Check sheet for the modelled part. Datum: model origin and axes. Units: mm. A direction names the side the tool comes from. Round coordinates to 2 decimals unless told otherwise and drop trailing zeros. Write each loop counter-clockwise with the first axis right and the second up, starting at its lowest first coordinate (ties: lowest second). Pieces come first, ordered by that corner, then holes. Notation, with made-up numbers: (-27, 9.25) -> (23, 9.25) arc R32 ccw to (23, 38.25) -> close; hole circle Ø5 at (87, 73.5). An arc over 180 degrees is marked (long way). Answer as a JSON object with one key per item and string values. Group by question number.
```python
from build123d import *

# Parameters (mm, degrees)
SCHIZZO1_R                   = 3
ESTRUSIONE_ESTRUSIONE1_DEPTH = 14
SMUSSO1_SIZE                 = 1
SCHIZZO6_R                   = 5
ESTRUSIONE_ESTRUSIONE3_DEPTH = 6
TAGLIO_ESTRUSIONE3_DEPTH     = 3
SCHIZZO8_R                   = 2.886751346
TAGLIO_ESTRUSIONE4_DEPTH     = 1
TAGLIO_ESTRUSIONE4_TAPER     = 45
RACCORDO1_R                  = 0.5
SCHIZZO9_R                   = 6
SCHIZZO9_R_2                 = 5
ESTRUSIONE_ESTRUSIONE4_DEPTH = 0.8
RACCORDO3_R                  = 0.1


with BuildPart() as part:
    # Schizzo1 → Estrusione-Estrusione1 (new body)
    with BuildSketch(Plane.XY):
        Circle(SCHIZZO1_R)
    extrude(amount=ESTRUSIONE_ESTRUSIONE1_DEPTH)

    # Smusso1
    smusso1_edges = [part.edges().sort_by_distance(p)[0] for p in [
        (-3, 0, 0),
    ]]
    chamfer(smusso1_edges, length=SMUSSO1_SIZE)

    # Schizzo6 → Estrusione-Estrusione3 (add)
    with BuildSketch(Plane.XY.offset(14)):
        Circle(SCHIZZO6_R)
    extrude(amount=ESTRUSIONE_ESTRUSIONE3_DEPTH)

    # Schizzo7 → Taglio-Estrusione3 (cut)
    with BuildSketch(Plane.XY.offset(20)):
        Polygon((1.443375673, 2.5), (-1.443375673, 2.5), (-2.886751346, 0), (-1.443375673, -2.5), (1.443375673, -2.5), (2.886751346, 0), align=None)
    extrude(amount=-TAGLIO_ESTRUSIONE3_DEPTH, mode=Mode.SUBTRACT)

    # Schizzo8 → Taglio-Estrusione4 (cut)
    with BuildSketch(Plane.XY.offset(20)):
        Circle(SCHIZZO8_R)
    extrude(amount=-TAGLIO_ESTRUSIONE4_DEPTH, taper=TAGLIO_ESTRUSIONE4_TAPER, mode=Mode.SUBTRACT)

    # Raccordo1
    raccordo1_edges = [part.edges().sort_by_distance(p)[0] for p in [
        (-5, 0, 20),
    ]]
    fillet(raccordo1_edges, radius=RACCORDO1_R)

    # Schizzo9 → Estrusione-Estrusione4 (add)
    with BuildSketch(Plane(origin=(0, 0, 14), x_dir=(-1, 0, 0), z_dir=(0, 0, -1))):
        Circle(SCHIZZO9_R)
        Circle(SCHIZZO9_R_2, mode=Mode.SUBTRACT)
    extrude(amount=-ESTRUSIONE_ESTRUSIONE4_DEPTH)

    # Raccordo3
    raccordo3_edges = [part.edges().sort_by_distance(p)[0] for p in [
        (-5, 0, 14.8),
        (6, 0, 14.8),
        (6, 0, 14),
    ]]
    fillet(raccordo3_edges, radius=RACCORDO3_R)


solid = part.part
```
(1) Access from +Z, -Z, +X, -X, +Y, -Y to the whole of each face (thin tool, end or side, straight path). Record for faces 4 (the flat face through (0, 0, 17)), 5 (the cylindrical face through (5.994, 0.264, 14.396)), 6 (the flat face through (3, 1, 14)).
(2) Section check B-B on z = 12. Record the cut outline in (x, y).
(3) Release check for a two-part mould opening along Y. For faces 1 (the cylindrical face through (-3, 0, 7)), 2 (the flat face through (0, 0, 0)), 3 (the conical face through (-2.32, 1.36, 19.8)) record: pulls with the +Y half, pulls with the -Y half, needs draft (parallel to the pull), parting line crosses it, or undercut.
(4) Section check A-A on x = 0. Record the cut outline in (y, z), then the cut area to 3 significant figures.
(5) Go/stop test with flat-tipped pins: pin 1 Ø1.5 at (x, y) = (-1, 0.5) entering from +Z; pin 2 Ø2 at (y, z) = (3.5, 8) entering from -X; pin 3 Ø0.9 at (x, z) = (0, 18.5) entering from -Y. Record where each tip stops, or that it passes through.
(6) Scan lines: line 1 along Z through (x, y) = (-2.5, -3); line 2 along Z through (x, y) = (5.75, 0.5); line 3 along Y through (x, z) = (0, 8.5). Record each from-to range of solid material in increasing order.
(7) Section check C-C on z = 16. Record the cut outline in (x, y).
Data:
{
 "1": {"face 4": "+Z", "face 5": "+Z, -Z", "face 6": "-Z"},
 "2": {"outline": "circle Ø6 at (0, 0)"},
 "3": {"face 1": "parting line crosses it", "face 2": "needs draft", "face 3": "undercut"},
 "4": {"outline": "(-6, 14.1) arc R0.1 ccw to (-5.9, 14) -> (-3, 14) -> (-3, 1) -> (-2, 0) -> (2, 0) -> (3, 1) -> (3, 14) -> (5.9, 14) arc R0.1 ccw to (6, 14.1) -> (6, 14.7) arc R0.1 ccw to (5.9, 14.8) -> (5.1, 14.8) arc R0.1 cw to (5, 14.9) -> (5, 19.5) arc R0.5 ccw to (4.5, 20) -> (2.89, 20) -> (2.5, 19.61) -> (2.5, 17) -> (-2.5, 17) -> (-2.5, 19.61) -> (-2.89, 20) -> (-4.5, 20) arc R0.5 ccw to (-5, 19.5) -> (-5, 14.9) arc R0.1 cw to (-5.1, 14.8) -> (-5.9, 14.8) arc R0.1 ccw to (-6, 14.7) -> close", "area": "129 mm²"},
 "5": {"pin 1": "stops at z = 17", "pin 2": "stops at x = -1.66", "pin 3": "stops at y = -5"},
 "6": {"line 1": "z = 14 to 20", "line 2": "z = 14 to 14.8", "line 3": "y = -3 to 3"},
 "7": {"outline": "circle Ø10 at (0, 0)"}
}
